from build123d import *

# Parameters (mm, degrees)
SKETCH1_W                   = 31.75
SKETCH1_H                   = 31.75
BOSS_EXTRUDE1_DEPTH         = 3.175
F_1_4_20_TAPPED_HOLE1_D     = 5.1054
F_1_4_20_TAPPED_HOLE1_DEPTH = 16.51
F_1_4_20_TAPPED_HOLE1_TIP   = 1.533816902


with BuildPart() as part:
    # Sketch1 → Boss-Extrude1 (new body)
    with BuildSketch(Plane(origin=(0, 0, 0), x_dir=(1, 0, 0), z_dir=(0, 1, 0))):
        with Locations((15.875, 15.875)):
            Rectangle(SKETCH1_W, SKETCH1_H)
    extrude(amount=BOSS_EXTRUDE1_DEPTH)

    # 1/4-20 Tapped Hole1
    with Locations(Plane(origin=(0, 3.175, 0), x_dir=(1, 0, 0), z_dir=(0, 1, 0))):
        with Locations((15.875, 15.875)):
            Hole(F_1_4_20_TAPPED_HOLE1_D / 2, depth=F_1_4_20_TAPPED_HOLE1_DEPTH)
            with Locations((0, 0, -(F_1_4_20_TAPPED_HOLE1_DEPTH + F_1_4_20_TAPPED_HOLE1_TIP / 2))):  # 118° drill point
                Cone(0, F_1_4_20_TAPPED_HOLE1_D / 2, F_1_4_20_TAPPED_HOLE1_TIP, mode=Mode.SUBTRACT)


solid = part.part
The listing builds one solid part. Answer for the finished solid, in the listing's coordinates (mm). Give positions to 0.01 mm unless a question says otherwise; leave off trailing zeros. Loops run counter-clockwise (first coordinate to the right, second up) from the corner with the lowest first, then second, coordinate; pieces in that order, holes last. Notation, with made-up numbers: (37, 15.5) - (81, 15.5) arc R15 ccw to (81, 35.5) - close; hole circle Ø9 at (44.25, 81). An arc over 180 degrees is marked (long way). Use one line per item in the form item = value.
1. The mould has two halves that part along X. Classify faces 1 (the face through (14.503, 1.565, -18.027)), 2 (the face through (0, 2, -16)), 3 (the face through (12, 0, -16)): pulls with the +X half, pulls with the -X half, needs draft (parallel to the pull), parting line crosses it, or undercut.
Calculated:
face_1 = undercut
face_2 = pulls with the -X half
face_3 = needs draft
2. Section B-B on z = -17 is taken. Give the vertices of the cut face in (x, y) (3 decimals).
Calculated:
outline = (0, 0) - (13.584, 0) - (13.584, 3.175) - (0, 3.175) - close; (18.166, 0) - (31.75, 0) - (31.75, 3.175) - (18.166, 3.175) - close
3. Section C-C on y = 1.65 is taken. Give the vertices of the cut face in (x, z) (3 decimals).
Calculated:
outline = (0, -31.75) - (31.75, -31.75) - (31.75, 0) - (0, 0) - close; hole circle Ø5.105 at (15.875, -15.875)
4. Section A-A on x = 17 is taken. Give the vertices of the cut face in (y, z) (3 decimals), then the cut area to 3 significant figures.
Calculated:
outline = (0, -31.75) - (3.175, -31.75) - (3.175, -18.166) - (0, -18.166) - close; (0, -13.584) - (3.175, -13.584) - (3.175, 0) - (0, 0) - close
area = 86.3 mm^2
5. Find the intervals of material crossed by line 1 along X through (y, z) = (2.35, -16); line 2 along Z through (x, y) = (16, 0.7); line 3 along X through (y, z) = (0.35, -14), in increasing order. Write a range as [from, to].
Calculated:
line_1 = [0, 13.33], [18.42, 31.75]
line_2 = [-31.75, -18.42], [-13.33, 0]
line_3 = [0, 14.14], [17.61, 31.75]
